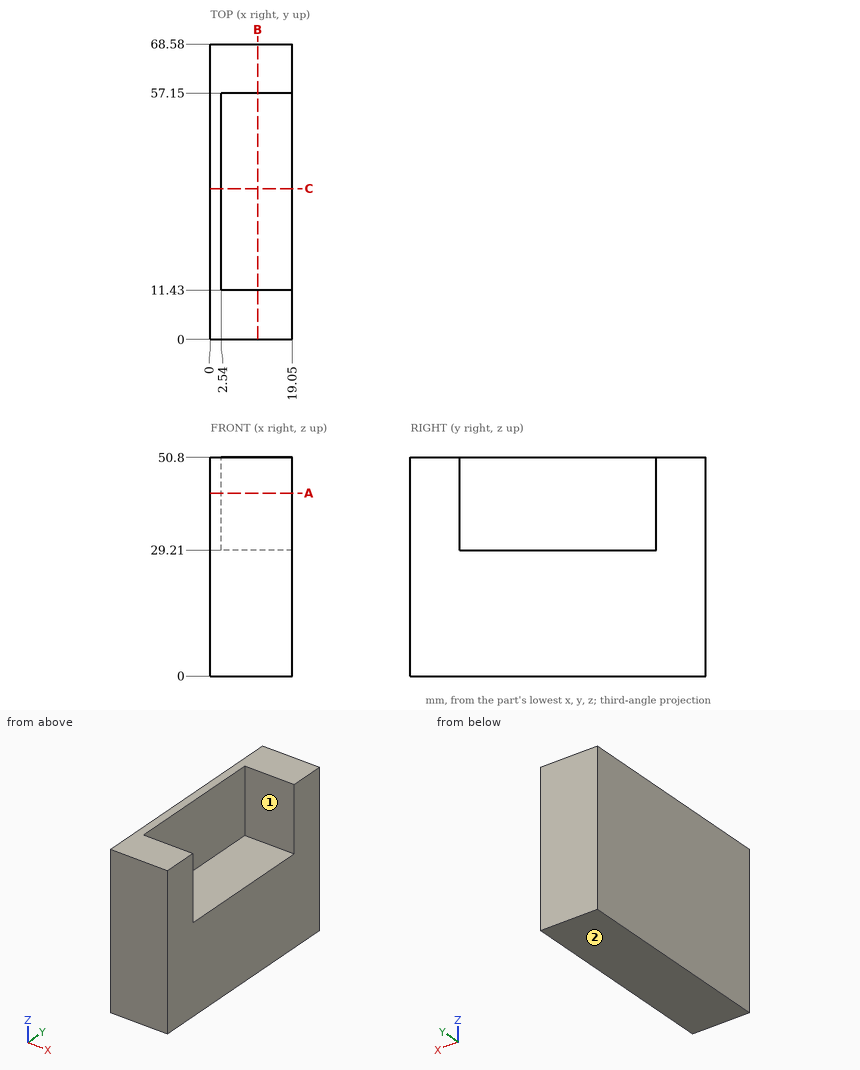
Part print with two shaded views. Sizes in mm from the minimum x, y, z corner. A direction names the side the tool comes from. Coordinates: 2 decimals unless noted, no trailing zeros. Order: outer loops, then holes, each group sorted by start corner. A loop starts at its lowest first (then second) coordinate and runs counter-clockwise, first axis right, second up.
(1) Drill centre lines: L1, parallel to Y at x = 10, z = 41; L2, parallel to Z at x = 7.5, y = 34; L3, parallel to X at y = 33, z = 31.5. Where is each one in solid material? Low to high.
Solution:
L1: y = 0 to 11.43, 57.15 to 68.58
L2: z = 0 to 29.21
L3: x = 0 to 2.54
(2) Saw through at B-B, the plane x = 11. Write the cut outline in (y, z), and give its area (3 significant figures).
Solution:
outline: (0, 0) - (68.58, 0) - (68.58, 50.8) - (57.15, 50.8) - (57.15, 29.21) - (11.43, 29.21) - (11.43, 50.8) - (0, 50.8) - close
area: 2,500 mm2
(3) Saw through at C-C, the plane y = 35. Write the cut outline in (x, z).
Solution:
outline: (0, 0) - (19.05, 0) - (19.05, 29.21) - (2.54, 29.21) - (2.54, 50.8) - (0, 50.8) - close
(4) Saw through at A-A, the plane z = 42.5. Write the cut outline in (x, y), and give its area (3 significant figures).
Solution:
outline: (0, 0) - (19.05, 0) - (19.05, 11.43) - (2.54, 11.43) - (2.54, 57.15) - (19.05, 57.15) - (19.05, 68.58) - (0, 68.58) - close
area: 552 mm2
(5) Which spindle directions (+Z, -Z, +X, -X, +Y, -Y) get a long thin tool onto all of the face, cutting with end or side? Do the marked faces 1 and 2. Say none if no direction does.
Solution:
face 1: +Z, +X
face 2: -Z, +X, -X, +Y, -Y
(6) Pin check, flat tips, straight feed: pin 1 Ø8 at (y, z) = (43, 33.5) entering from +X; pin 2 Ø3 at (x, y) = (4, 28) entering from -Z; pin 3 Ø1.5 at (x, y) = (8, 56) entering from +Z. Stop position of each tip, or through.
Solution:
pin 1: stops at x = 2.54
pin 2: stops at z = 0
pin 3: stops at z = 29.21
